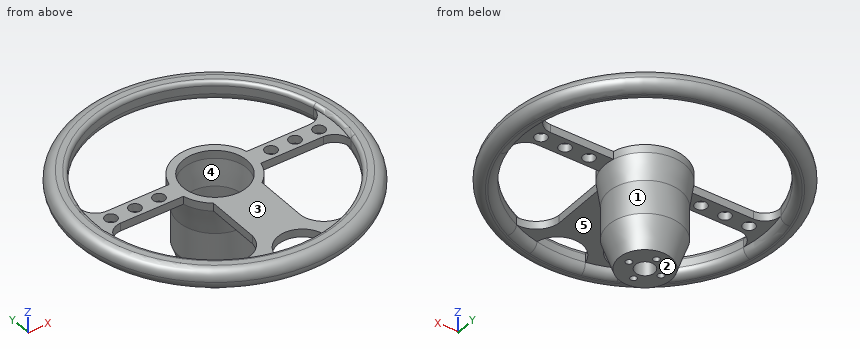
from build123d import *

# Parameters (mm, degrees)
SZKIC1_R                    = 175
SZKIC1_R_2                  = 40
SZKIC1_R_3                  = 7.5
DODANIE_WYCI_GNI_CIE1_DEPTH = 25
ZAOKR_GLENIE1_R             = 12.5
SZKIC2_W                    = 10
SZKIC2_H                    = 150
SZKIC3_W                    = 5
SZKIC3_H                    = 150
ZAOKR_GLENIE4_R             = 10
ZAOKR_GLENIE5_R             = 5
SZKIC5_R                    = 12
SZKIC5_R_2                  = 4
WYTNIJ_WYCI_GNI_CIE1_DEPTH  = 25
DODANIE_WYCI_GNI_CIE4_START = 45
SZKIC9_R                    = 27.052132897
SZKIC9_R_2                  = 12
SZKIC9_R_3                  = 4
DODANIE_WYCI_GNI_CIE4_DEPTH = 45


with BuildPart() as part:
    # Szkic1 → Dodanie-wyciągnięcie1 (new body)
    with BuildSketch(Plane.XY):
        Circle(SZKIC1_R)
        Circle(SZKIC1_R_2, mode=Mode.SUBTRACT)
        with BuildLine():
            ThreePointArc((63.948658552, -135.685552176), (41.3963046, -128.857575517), (30.277490786, -108.082544509))
            Line((30.277490786, -108.082544509), (30.277490786, -39.790370088))
            ThreePointArc((30.277490786, -39.790370088), (41.668308443, -27.636064689), (48.434312767, -12.414400782))
            Line((48.434312767, -12.414400782), (126.821344913, -12.414400782))
            ThreePointArc((126.821344913, -12.414400782), (140.806039181, -18.492039568), (146.397171731, -32.678251316))
            ThreePointArc((146.397171731, -32.678251316), (117.106652616, -93.733835476), (63.948658552, -135.685552176))
        make_face(mode=Mode.SUBTRACT)
        with BuildLine():
            ThreePointArc((146.397171731, 32.678251316), (140.806039181, 18.492039568), (126.821344913, 12.414400782))
            Line((126.821344913, 12.414400782), (48.434312767, 12.414400782))
            ThreePointArc((48.434312767, 12.414400782), (0, 50), (-48.434312767, 12.414400782))
            Line((-48.434312767, 12.414400782), (-126.821344913, 12.414400782))
            ThreePointArc((-126.821344913, 12.414400782), (-140.806039181, 18.492039568), (-146.397171731, 32.678251316))
            ThreePointArc((-146.397171731, 32.678251316), (0, 150), (146.397171731, 32.678251316))
        make_face(mode=Mode.SUBTRACT)
        with BuildLine():
            ThreePointArc((-146.397171731, -32.678251316), (-140.806039181, -18.492039568), (-126.821344913, -12.414400782))
            Line((-126.821344913, -12.414400782), (-48.434312767, -12.414400782))
            ThreePointArc((-48.434312767, -12.414400782), (-41.668308443, -27.636064689), (-30.277490786, -39.790370088))
            Line((-30.277490786, -39.790370088), (-30.277490786, -108.082544509))
            ThreePointArc((-30.277490786, -108.082544509), (-41.3963046, -128.857575517), (-63.948658552, -135.685552176))
            ThreePointArc((-63.948658552, -135.685552176), (-117.106652616, -93.733835476), (-146.397171731, -32.678251316))
        make_face(mode=Mode.SUBTRACT)
        with BuildLine():
            ThreePointArc((-30.277490786, -146.912469014), (0, -122.410388377), (30.277490786, -146.912469014))
            ThreePointArc((30.277490786, -146.912469014), (0, -150), (-30.277490786, -146.912469014))
        make_face(mode=Mode.SUBTRACT)
        with Locations((-70, 0)):
            Circle(SZKIC1_R_3, mode=Mode.SUBTRACT)
        with Locations((-100, 0)):
            Circle(SZKIC1_R_3, mode=Mode.SUBTRACT)
        with Locations((-130, 0)):
            Circle(SZKIC1_R_3, mode=Mode.SUBTRACT)
        with Locations((100, 0)):
            Circle(SZKIC1_R_3, mode=Mode.SUBTRACT)
        with Locations((70, 0)):
            Circle(SZKIC1_R_3, mode=Mode.SUBTRACT)
        with Locations((130, 0)):
            Circle(SZKIC1_R_3, mode=Mode.SUBTRACT)
    extrude(amount=DODANIE_WYCI_GNI_CIE1_DEPTH)

    # Zaokrąglenie1
    zaokr_glenie1_edges = [part.edges().sort_by_distance(p)[0] for p in [
        (-175, 0, 25),
        (-175, 0, 0),
    ]]
    fillet(zaokr_glenie1_edges, radius=ZAOKR_GLENIE1_R - 0.0001)  # a hair under: the kernel refuses the full size

    # Szkic2 → Wycięcie-obrót1 (revolve, cut)
    with BuildSketch(Plane(origin=(0, 0, 0), x_dir=(0, 0, -1), z_dir=(1, 0, 0)), mode=Mode.PRIVATE) as wyci_cie_obr_t1_sk:
        with Locations((-5, -75)):
            Rectangle(SZKIC2_W, SZKIC2_H)
    revolve(wyci_cie_obr_t1_sk.sketch.rotate(Axis((0, 0, 10), (0, 0, -1)), 77.416921492), axis=Axis((0, 0, 10), (0, 0, -1)), mode=Mode.SUBTRACT)

    # Szkic3 → Wycięcie-obrót2 (revolve, cut)
    with BuildSketch(Plane(origin=(0, 0, 0), x_dir=(0, 0, -1), z_dir=(1, 0, 0)), mode=Mode.PRIVATE) as wyci_cie_obr_t2_sk:
        with Locations((-22.5, -75)):
            Rectangle(SZKIC3_W, SZKIC3_H)
    revolve(wyci_cie_obr_t2_sk.sketch.rotate(Axis((0, 0, 20), (0, 0, 1)), 90), axis=Axis((0, 0, 20), (0, 0, 1)), mode=Mode.SUBTRACT)

    # Zaokrąglenie4
    zaokr_glenie4_edges = [part.edges().sort_by_distance(p)[0] for p in [
        (150, 0, 0),
    ]]
    fillet(zaokr_glenie4_edges, radius=ZAOKR_GLENIE4_R - 0.0001)  # a hair under: the kernel refuses the full size

    # Zaokrąglenie5
    zaokr_glenie5_edges = [part.edges().sort_by_distance(p)[0] for p in [
        (149.096572328, -16.438130069, 25),
    ]]
    fillet(zaokr_glenie5_edges, radius=ZAOKR_GLENIE5_R - 0.0001)  # a hair under: the kernel refuses the full size

    # Szkic4 → Obrót3 (revolve)
    with BuildSketch(Plane(origin=(0, 0, 0), x_dir=(0, 0, -1), z_dir=(1, 0, 0))):
        Polygon((-10, 50), (21.913455258, 45.379893009), (63.909884625, 45.379893009), (100.428518858, 32.678251316), (100.428518858, 0), (90.618518858, 0), (90.618518858, 27.052132897), (63.909884625, 35.565510059), (21.913455258, 35.565510059), (-10, 40), align=None)
    revolve(axis=Axis((0, 0, -90.618518858), (0, 0, 1)))

    # Szkic5 → Wytnij-wyciągnięcie1 (cut)
    with BuildSketch(Plane.XY.offset(-90.618518858)):
        Circle(SZKIC5_R)
        with Locations((0, 20)):
            Circle(SZKIC5_R_2)
        with Locations((20, 0)):
            Circle(SZKIC5_R_2)
        with Locations((0, -20)):
            Circle(SZKIC5_R_2)
        with Locations((-20, 0)):
            Circle(SZKIC5_R_2)
    extrude(amount=-WYTNIJ_WYCI_GNI_CIE1_DEPTH, mode=Mode.SUBTRACT)

    # Szkic9 → Dodanie-wyciągnięcie4 (add)
    with BuildSketch(Plane.XY.offset(-90.618518858).offset(DODANIE_WYCI_GNI_CIE4_START)):
        with Locations(Location((0, 0, 0), (0, 0, 180))):
            Circle(SZKIC9_R)
        Circle(SZKIC9_R_2, mode=Mode.SUBTRACT)
        with Locations((0, 20)):
            Circle(SZKIC9_R_3, mode=Mode.SUBTRACT)
        with Locations((20, 0)):
            Circle(SZKIC9_R_3, mode=Mode.SUBTRACT)
        with Locations((0, -20)):
            Circle(SZKIC9_R_3, mode=Mode.SUBTRACT)
        with Locations((-20, 0)):
            Circle(SZKIC9_R_3, mode=Mode.SUBTRACT)
    extrude(amount=-DODANIE_WYCI_GNI_CIE4_DEPTH)

    # Szkic10 → Obrót4 (revolve)
    with BuildSketch(Plane(origin=(0, 0, 0), x_dir=(0, 0, -1), z_dir=(1, 0, 0)), mode=Mode.PRIVATE) as obr_t4_sk:
        Polygon((63.909884625, 35.565510059), (45.618518858, 35.565510059), (45.618518858, 12), (57.670604535, 12), (57.670604535, 27.052132897), (90.618518858, 27.052132897), align=None)
    revolve(obr_t4_sk.sketch.rotate(Axis((0, 0, 0), (0, 0, -1)), 90), axis=Axis((0, 0, 0), (0, 0, -1)))


solid = part.part
Here's how the part is built. I have some questions about the finished solid (model axes, mm). Face numbers are marked on the shaded views. A direction names the side the tool comes from. Round coordinates to 2 decimals unless told otherwise and drop trailing zeros. Write each loop counter-clockwise with the first axis right and the second up, starting at its lowest first coordinate (ties: lowest second). Pieces come first, ordered by that corner, then holes. Notation, with made-up numbers: (17, 13) -> (60, 13) arc R21 ccw to (60, 43) -> close; hole circle Ø7 at (81, 32). An arc over 180 degrees is marked (long way). One line per item, written item: value.
1) Suppose I cut it at C-C on z = -79. List the corners of the cut face in (x, y) for me.
Filled sheet:
outline: circle Ø80.26 at (0, 0); hole circle Ø8 at (-20, 0); hole circle Ø24 at (0, 0); hole circle Ø8 at (0, -20); hole circle Ø8 at (0, 20); hole circle Ø8 at (20, 0)
2) If I drill on line 1 (Y direction, x = -100, z = 17.5); line 2 (Y direction, x = 0, z = -88); line 3 (X direction, y = 41.5, z = 7.5), over which ranges is the centre line in solid material (lowest first)? Write a range as [from, to].
Filled sheet:
line 1: y = [-142.34, -111.8], [-12.41, -7.5], [7.5, 12.41], [111.8, 142.34]
line 2: y = [-37, -24], [-16, -12], [12, 16], [24, 37]
line 3: x = [-168.93, -144.48], [-27.23, 27.23], [144.48, 168.93]
3) We'd pull the mould along X, two halves only. Please class the marked faces 1, 2 and 3: released by +X, released by -X, zero draft, split by the parting line, or undercut.
Filled sheet:
face 1: split by the parting line
face 2: zero draft
face 3: undercut
4) Suppose I cut it at A-A on z = -39.5. List the corners of the cut face in (x, y) for me.
Filled sheet:
outline: circle Ø90.76 at (0, 0); hole circle Ø71.13 at (0, 0)
5) I'm going to push flat-ended pins straight in: pin 1 Ø12 at (x, y) = (-100, 0) entering from +Z; pin 2 Ø5 at (x, y) = (20, 0) entering from +Z; pin 3 Ø2.5 at (x, y) = (-21, 0.5) entering from -Z; pin 4 Ø2 at (y, z) = (-36, -23.5) entering from +X. Where does each tip first touch, or does it pass through?
Filled sheet:
pin 1: passes through
pin 2: stops at z = -45.62
pin 3: stops at z = -57.67
pin 4: stops at x = 28.88
6) For the marked faces 4 and 5, which set-ups out of +Z, -Z, +X, -X, +Y, -Y let a thin tool reach every point of the face, with its end or its side?
Filled sheet:
face 4: +Z
face 5: -Z
7) Suppose I cut it at B-B on x = 100. Give the number of separate pieces and of enclosed holes in the cut face, plus the area to 3 significant figures.
Filled sheet:
separate pieces: 4
enclosed holes: 0
area: 1,450 mm2
